from build123d import *

# Parameters (mm, degrees)
BOSS_EXTRUDE1_DEPTH          = 3.175
F_1_8_0_125_DIAMETER_HOLE1_D = 3.175
SKETCH6_R                    = 12.7
CUT_EXTRUDE1_DEPTH           = 17.0815


with BuildPart() as part:
    # Sketch1 → Boss-Extrude1 (new body)
    with BuildSketch(Plane.XY):
        with BuildLine():
            Line((0, 107.95), (38.1, 107.95))
            Line((38.1, 107.95), (38.1, -107.95))
            Line((38.1, -107.95), (0, -107.95))
            ThreePointArc((0, -107.95), (-107.95, 0), (0, 107.95))
        make_face()
    extrude(amount=BOSS_EXTRUDE1_DEPTH)

    # 1/8 (0.125) Diameter Hole1 (through all)
    with Locations(Plane(origin=(0, 0, 0), x_dir=(-1, 0, 0), z_dir=(0, 0, -1))):
        with Locations((12.262546259, -20.412376527), (0, 95.25), (0, -95.25), (0, -69.85), (0, 69.85), (0, 0), (23.808909754, 0.413488312), (11.546363494, 20.825864839), (-12.262546259, 20.412376527), (-23.808909754, -0.413488312), (-11.546363494, -20.825864839)):
            Hole(F_1_8_0_125_DIAMETER_HOLE1_D / 2)

    # Sketch6 → Cut-Extrude1 (cut)
    with BuildSketch(Plane(origin=(0, 0, 0), x_dir=(-1, 0, 0), z_dir=(0, 0, -1))):
        Circle(SKETCH6_R)
    extrude(amount=-CUT_EXTRUDE1_DEPTH, mode=Mode.SUBTRACT)


solid = part.part
Input: part model. Units: mm. Frame: model coordinates. Coordinates: 2 decimals unless noted, no trailing zeros. Loops run counter-clockwise (first coordinate to the right, second up) from the corner with the lowest first, then second, coordinate; pieces in that order, holes last. Notation, with made-up numbers: (81, 65.5) - (140, 65.5) arc R20 ccw to (140, 91.5) - close; hole circle Ø8 at (50, -6). An arc over 180 degrees is marked (long way). Answer in a Markdown table with one row per item. Add a question column.
Item 1: Section query C-C on x = -67.5. Return the cut outline in (y, z) (3 decimals).
Item 2: Section query A-A on z = 1.45. State how many separate pieces and enclosed holes the cut face has, then the cut area to 3 significant figures.
Item 3: Mould query, pull axis X, two halves, no side actions, for faces 1 (the cylindrical face through (-107.924, -2.374, 1.565)), 2 (the flat face through (-18, 2, 3.175)), 3 (the cylindrical face through (2.75, -12.4, 1.57)). Classes: released by +X, released by -X, zero draft, split by the parting line, or undercut.
Item 4: Section query B-B on y = 56.5. Return the cut outline in (x, z) (3 decimals).
Item 5: Line query: line 1 along Y through (x, z) = (0, 2); line 2 along X through (y, z) = (-21.5, 1.9); line 3 along Y through (x, z) = (-1, 1.1). Output: solid intervals per line, ascending. Write a range as [from, to].
Item 6: Contact query for flat-ended pins moving along their axis: P1, Ø3, axis at x = 11.55, y = -20.83, coming from the -Z side; P2, Ø1, axis at y = 55.5, z = 1, coming from the -X side. Output: stop coordinate, or through.
Recorded:
| question | item | result |
|---|---|---|
| 1 | outline | (-84.243, 0) - (84.243, 0) - (84.243, 3.175) - (-84.243, 3.175) - close |
| 2 | separate pieces | 1 |
| 2 | enclosed holes | 11 |
| 2 | area | 25,900 mm^2 |
| 3 | face 1 | released by -X |
| 3 | face 2 | zero draft |
| 3 | face 3 | undercut |
| 4 | outline | (-91.983, 0) - (38.1, 0) - (38.1, 3.175) - (-91.983, 3.175) - close |
| 5 | line 1 | [-107.95, -96.84], [-93.66, -71.44], [-68.26, -12.7], [12.7, 68.26], [71.44, 93.66], [96.84, 107.95] |
| 5 | line 2 | [-105.79, -13.42], [-11.11, 10.11], [12.98, 38.1] |
| 5 | line 3 | [-107.95, -96.48], [-94.02, -71.08], [-68.62, -12.66], [12.66, 68.62], [71.08, 94.02], [96.48, 107.95] |
| 6 | P1 | through |
| 6 | P2 | x = -92.89 |
